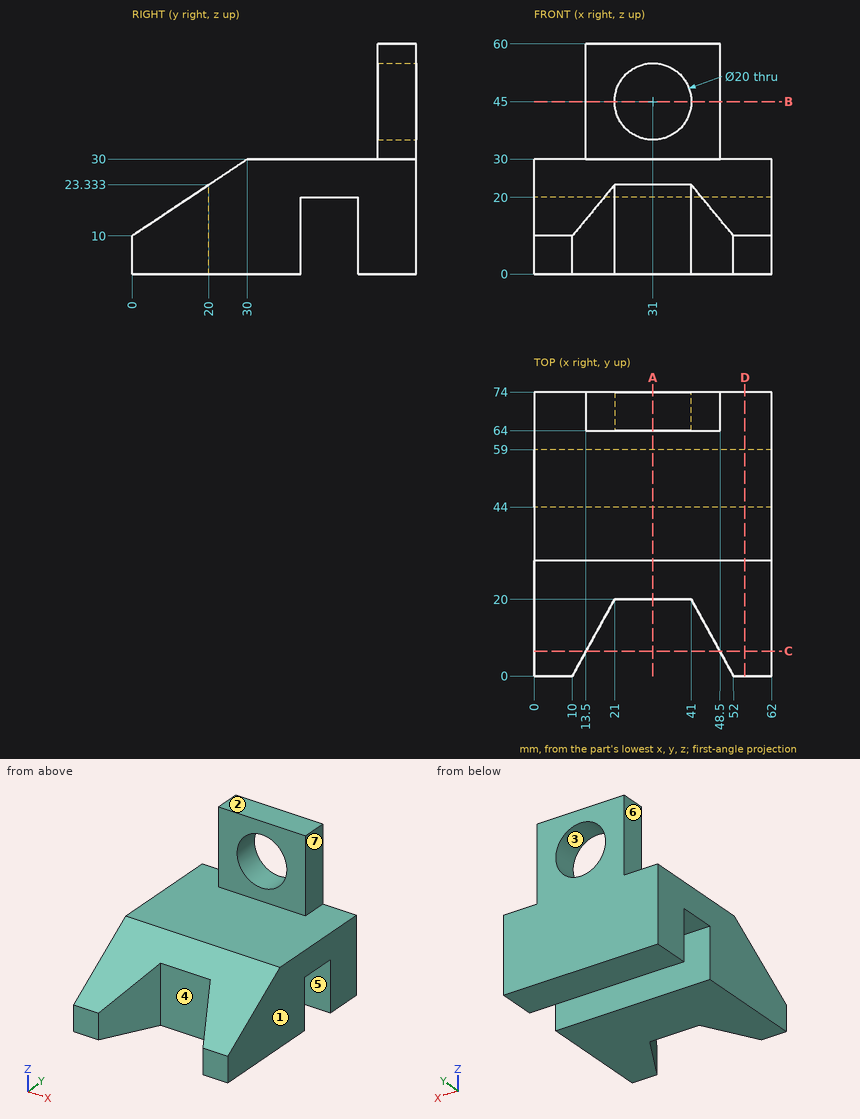
Can you work these out from the drawing? Everything is in mm from the part's minimum corner. A direction names the side the tool comes from. Round coordinates to 2 decimals unless told otherwise and drop trailing zeros. Loops run counter-clockwise (first coordinate to the right, second up) from the corner with the lowest first, then second, coordinate; pieces in that order, holes last.
1. If we section it at A-A on x = 31: Write out the boundary of the cut face in (y, z).
Answer list:
outline: (20, 0) - (44, 0) - (44, 20) - (59, 20) - (59, 0) - (74, 0) - (74, 35) - (64, 35) - (64, 30) - (30, 30) - (20, 23.33) - close; (64, 55) - (74, 55) - (74, 60) - (64, 60) - close
2. We'd pull the mould along X, two halves only. Please class the marked faces 1, 2 and 3: +X half, -X half, draft (parallel to the pull), parting line (faces both ways), or undercut.
Answer list:
face 1: +X half
face 2: draft
face 3: undercut
3. Which directions (+Z, -Z, +X, -X, +Y, -Y) give clear straight access to the entire face, cutting with the end or side of a thin tool? Please do the marked faces 4, 5, 6 and 7.
Answer list:
face 4: +Z, -Z, -Y
face 5: -Z, +X, -X
face 6: +Z, -X, +Y, -Y
face 7: +Z, +X, +Y, -Y
4. If we section it at D-D on x = 55: Write out the boundary of the cut face in (y, z), plus the area to 3 significant figures.
Answer list:
outline: (0, 0) - (44, 0) - (44, 20) - (59, 20) - (59, 0) - (74, 0) - (74, 30) - (30, 30) - (0, 10) - close
area: 1,620 mm2
5. If we section it at C-C on y = 6.5: Write out the boundary of the cut face in (x, z) (1 decimal), plus the area to 3 significant figures.
Answer list:
outline: (0, 0) - (13.6, 0) - (13.6, 14.3) - (0, 14.3) - close; (48.4, 0) - (62, 0) - (62, 14.3) - (48.4, 14.3) - close
area: 389 mm2
6. If we section it at B-B on z = 45: Write out the boundary of the cut face in (x, y).
Answer list:
outline: (13.5, 64) - (21, 64) - (21, 74) - (13.5, 74) - close; (41, 64) - (48.5, 64) - (48.5, 74) - (41, 74) - close
7. If I drill on line 1 along Z through (x, y) = (31, 67.25); line 2 along Y through (x, z) = (52, 5); line 3 along Y through (x, z) = (14.5, 11.5), over which ranges is the centre line in solid material (lowest first)?
Answer list:
line 1: z = 0 to 35, 55 to 60
line 2: y = 0 to 44, 59 to 74
line 3: y = 8.18 to 44, 59 to 74
8. For P1, Ø10, axis at x = 45, z = 9.5, coming from the -Y side (1 decimal); P2, Ø4, axis at x = 38, z = 18.5, coming from the -Y side; P3, Ø23, axis at x = 31, z = 45, coming from the -Y side, each with a flat end and sliding along its axis, tell me the tip position at first contact or that it passes through.
Answer list:
P1: stops at y = 3.6
P2: stops at y = 20
P3: stops at y = 64
